The listing builds one solid part. Answer for the finished solid, in the listing's coordinates (mm). A direction names the side the tool comes from. Coordinates: 2 decimals unless noted, no trailing zeros. Loops run counter-clockwise (first coordinate to the right, second up) from the corner with the lowest first, then second, coordinate; pieces in that order, holes last. Notation, with made-up numbers: (-29, -12) - (1, -12) arc R11 ccw to (1, -3) - close; hole circle Ø2 at (74, -37.75). An arc over 180 degrees is marked (long way). Return JSON: item names as keys, results as strings. Group by question number.
1. Section C-C (y = 58) is taken. Write down the section's boundary in (x, z).
2. Section B-B (z = 0) is taken. Write down the section's boundary in (x, y), and give its area (3 significant figures).
3. Find the intervals of material crossed by line 1 along Y through (x, z) = (6, 37.5); line 2 along X through (y, z) = (42, 0); line 3 along X through (y, z) = (-14.5, -9), in increasing order.
4. Section D-D (y = 18.5) is taken. Write down the section's boundary in (x, z), and give its area (3 significant figures).
5. Section A-A (x = 0) is taken. Write down the section's boundary in (y, z).
6. Which of the six approach directions +Z, -Z, +X, -X, +Y, -Y give full straight-line access (tool end or side, diameter ignored) to faces 1 (the face through (12.7, 13, 48)), 2 (the face through (-12.7, 13, 48)), 3 (the face through (-2.75, -12.52, 12.4))?
7. Each of these flat-tipped pins is pushed along its axis until it touches: P1, Ø1, axis at x = 25.5, z = 31, coming from the -Y side; P2, Ø2.5, axis at y = 10, z = 48, coming from the -X side; P3, Ø2, axis at x = -21.5, z = -25.5, coming from the +Y side. Where does it stop, or does it pass through?
Autodesk Inventor part; units mm, degrees
ref_plane "YZ Plane" through (0, 0, 0) normal (1, 0, 0) x (0, 1, 0)
ref_plane "XZ Plane" through (0, 0, 0) normal (0, 1, 0) x (-1, 0, 0)
sketch "Sketch1" plane through (0, 0, 0) normal (0, 1, 0) x (-1, 0, 0)
  circle A0 centre (0, 0) radius 48.26
  dimension "d0" = 96.52
extrude "Extrusion1" add sketch "Sketch1" along normal blind 25.4
sketch "Sketch2" plane through (0, 25.4, 0) normal (0, 1, 0) x (1, 0, 0)
  circle A0 centre (0, 0) radius 12.7
  dimension "d3" = 25.4
extrude "Extrusion2" add sketch "Sketch2" along normal blind 50.8
sketch "Sketch3" plane through (0, 0, 0) normal (0, -1, 0) x (1, 0, 0)
  circle A0 centre (0, 0) radius 12.7
  circle A1 centre (0, 0) radius 12.7
extrude "Extrusion3" add sketch "Sketch3" along normal blind 25.4
ref_plane "Work Plane1" through (0, 0, 48.26) normal (0, 0, 1) x (1, 0, 0)
sketch "Sketch4" plane through (0, 0, 48.26) normal (0, 0, 1) x (1, 0, 0)
  line L0 (0, 0) -> (0, 25.4)
  line L1 (0, 0) -> (12.7, 0)
  line L2 (0, 0) -> (-12.7, 0)
  line L3 (12.7, 0) -> (12.7, 25.4)
  line L4 (12.7, 25.4) -> (-12.7, 25.4)
  line L5 (-12.7, 25.4) -> (-12.7, 0)
  line L6 (-48.26, 0) -> (48.26, 0)
  dimension "d9" = 12.7
  dimension "d10" = 25.4
  dimension "d11" = 12.7
extrude "Extrusion4" add sketch "Sketch4" along normal blind 1.27 and the other way blind 12.7
properties part number "T100 rough draft"
The answers:
{
 "1": {"outline": "circle Ø25.4 at (0, 0)"},
 "2": {"outline": "(-48.26, 0) - (-12.7, 0) - (-12.7, -25.4) - (12.7, -25.4) - (12.7, 0) - (48.26, 0) - (48.26, 25.4) - (12.7, 25.4) - (12.7, 76.2) - (-12.7, 76.2) - (-12.7, 25.4) - (-48.26, 25.4) - close", "area": "4,390 mm2"},
 "3": {"line 1": "y = 0 to 25.4", "line 2": "x = -12.7 to 12.7", "line 3": "x = -8.96 to 8.96"},
 "4": {"outline": "(-12.7, 46.56) arc R48.26 ccw (long way) to (12.7, 46.56) - (12.7, 49.53) - (-12.7, 49.53) - close", "area": "7,360 mm2"},
 "5": {"outline": "(-25.4, -12.7) - (0, -12.7) - (0, -48.26) - (25.4, -48.26) - (25.4, -12.7) - (76.2, -12.7) - (76.2, 12.7) - (25.4, 12.7) - (25.4, 49.53) - (0, 49.53) - (0, 12.7) - (-25.4, 12.7) - close"},
 "6": {"face 1": "+Z, +X, +Y, -Y", "face 2": "+Z, -X, +Y, -Y", "face 3": "-Y"},
 "7": {"P1": "stops at y = 0", "P2": "stops at x = -12.7", "P3": "stops at y = 25.4"}
}
